Answer from the drawing. Dimensions are ordinates in mm from the lowest x, y and z of the part. A direction names the side the tool comes from. Give positions to 0.01 mm unless a question says otherwise; leave off trailing zeros. Loops run counter-clockwise (first coordinate to the right, second up) from the corner with the lowest first, then second, coordinate; pieces in that order, holes last. Notation, with made-up numbers: (6, -31) -> (53, -31) arc R25 cw to (53, 0) -> close; hole circle Ø8 at (48, 29). An arc over 180 degrees is marked (long way). Return JSON: item names as keys, results as strings. Group by question number.
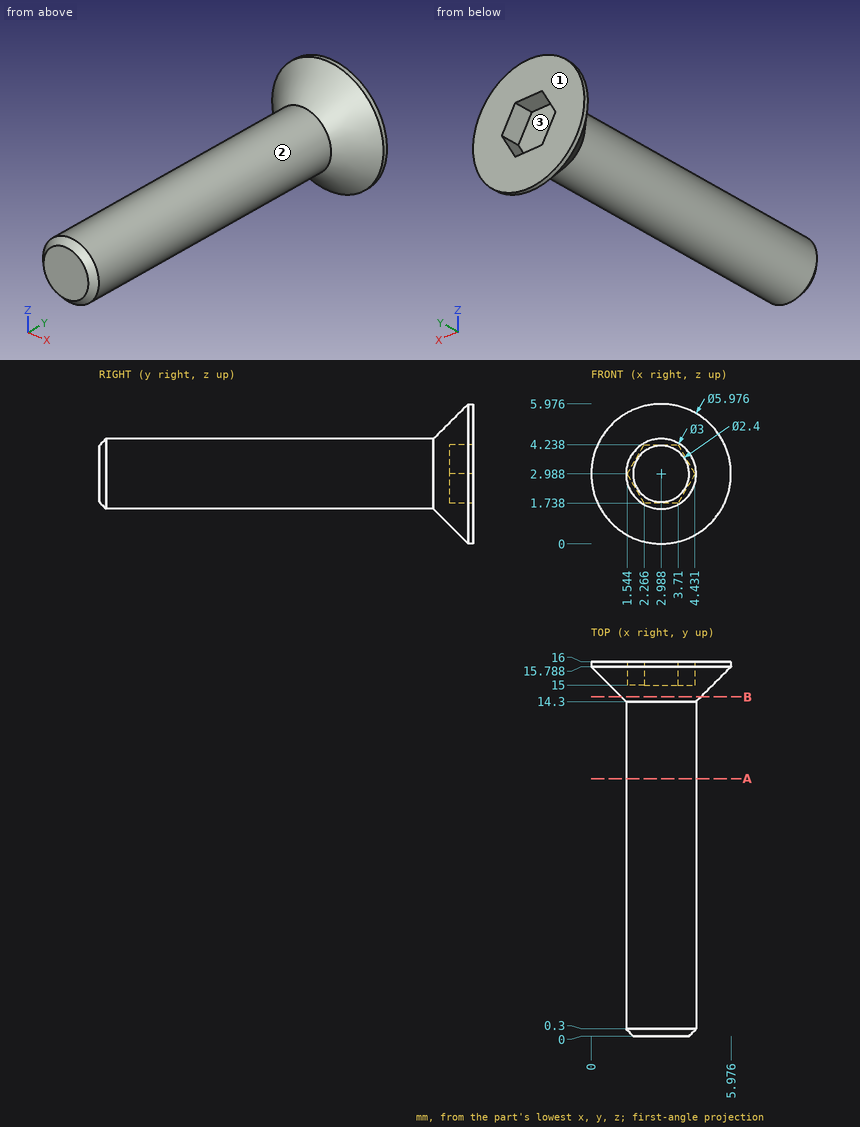
1. Straight lines are drawn through the part: line 1 (Y direction, x = 3.7, z = 2.95); line 2 (Z direction, x = 3.1, y = 11); line 3 (Y direction, x = 2.3, z = 1.55) (1 decimal). For each, find the intervals that lie inside material, in ascending order. Write a range as from..to.
2. Which of the six approach directions +Z, -Z, +X, -X, +Y, -Y give full straight-line access (tool end or side, diameter ignored) to the marked faces 1, 2 and 3?
3. Section A-A on y = 11 is taken. Determine the outline of the cut face in (x, z).
4. Section B-B on y = 14.5 is taken. Determine the outline of the cut face in (x, z).
5. Flat-ended cylindrical pins translate along their axes: pin 1 Ø3 at (x, z) = (1, 2.5) entering from -Y; pin 2 Ø2 at (x, y) = (1, 14) entering from +Z. Find the tip coordinate at first contact, or state that the pin passes through.
Completed:
{
 "1": {"line 1": "y = 0..15", "line 2": "z = 1.49..4.48", "line 3": "y = 14.4..16"},
 "2": {"face 1": "+Z, -Z, +X, -X, +Y", "face 2": "-Y", "face 3": "+Y"},
 "3": {"outline": "circle Ø3 at (2.99, 2.99)"},
 "4": {"outline": "circle Ø3.4 at (2.99, 2.99)"},
 "5": {"pin 1": "stops at y = 0", "pin 2": "stops at z = 4.43"}
}
